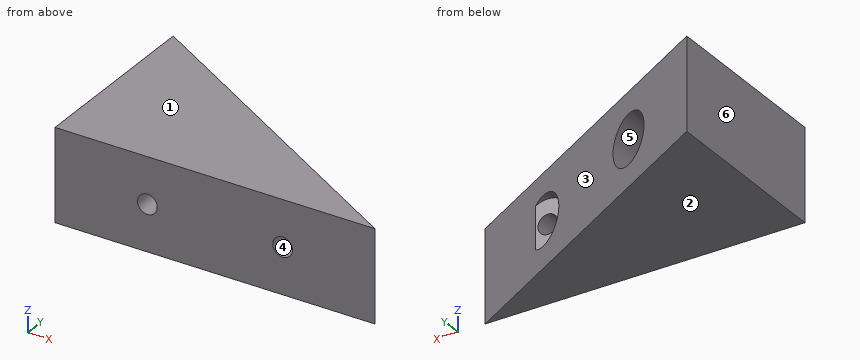
```python
from build123d import *

# Parameters (mm, degrees)
EXTRUDE_1_DEPTH          = 15
SKETCH_2_R               = 1.6
CUT_EXTRUDE_1_DEPTH      = 43.426406871
CUT_EXTRUDE_2_DEPTH      = 34.541019662
CUT_EXTRUDE_2_DEPTH_BACK = 7.5
SKETCH_3_R               = 4
SKETCH_3_R_2             = 1.6


with BuildPart() as part:
    # ｽｹｯﾁ1 → ﾎﾞｽ - 押し出し1 (new body)
    with BuildSketch(Plane.XY):
        Polygon((-25.980762114, 15), (-25.980762114, -15), (25.980762114, -15), align=None)
    extrude(amount=EXTRUDE_1_DEPTH)

    # ｽｹｯﾁ2 → ｶｯﾄ - 押し出し1 (cut, through all)
    with BuildSketch(Plane.XZ.offset(15)):
        with Locations(Location((-10.980762114, 7.5, 0), (0, 0, 270))):
            Circle(SKETCH_2_R)
        with Locations(Location((10.980762114, 7.5, 0), (0, 0, 270))):
            Circle(SKETCH_2_R)
    extrude(amount=-CUT_EXTRUDE_1_DEPTH, mode=Mode.SUBTRACT)

    # ｽｹｯﾁ3 → ｶｯﾄ - 押し出し2 (cut, two sides: drawn at the far end of the back side and taken through both)
    # profile 1 of 2: a face of its own
    with BuildSketch(Plane(origin=(0, 0, 0), x_dir=(1, 0, 0), z_dir=(0, 1, 0)).offset(-CUT_EXTRUDE_2_DEPTH_BACK)):
        with Locations((-10.980762114, -7.5)):
            Circle(SKETCH_3_R)
        with Locations(Location((-10.980762114, -7.5, 0), (0, 0, 90))):
            Circle(SKETCH_3_R_2, mode=Mode.SUBTRACT)
    # profile 2 of 2: a face of its own
    with BuildSketch(Plane(origin=(0, 0, 0), x_dir=(1, 0, 0), z_dir=(0, 1, 0)).offset(-CUT_EXTRUDE_2_DEPTH_BACK)):
        with Locations((10.980762114, -7.5)):
            Circle(SKETCH_3_R)
        with Locations(Location((10.980762114, -7.5, 0), (0, 0, 90))):
            Circle(SKETCH_3_R_2, mode=Mode.SUBTRACT)
    extrude(amount=CUT_EXTRUDE_2_DEPTH + CUT_EXTRUDE_2_DEPTH_BACK, mode=Mode.SUBTRACT)


solid = part.part
```
Check sheet for the modelled part. Datum: model origin and axes. Units: mm. Face numbers are marked on the shaded views. A direction names the side the tool comes from. Give positions to 0.01 mm unless a question says otherwise; leave off trailing zeros. Write each loop counter-clockwise with the first axis right and the second up, starting at its lowest first coordinate (ties: lowest second). Pieces come first, ordered by that corner, then holes.
Item 1: Cross-section at A-A (y = -10). Enter the section's corners in (x, z).
Item 2: Scan lines: L1, parallel to X at y = -10.5, z = 7.5; L2, parallel to X at y = -4.9, z = 7.5; L3, parallel to X at y = -11.75, z = 7.5. Record each from-to range of solid material in increasing order.
Item 3: Cross-section at D-D (x = -4.5). Enter the section's corners in (y, z), and give its area (3 significant figures).
Item 4: Access from +Z, -Z, +X, -X, +Y, -Y to the whole of each face (thin tool, end or side, straight path). Record for the marked faces 5 and 6.
Item 5: Cross-section at B-B (z = 7.5). Enter the section's corners in (x, y).
Item 6: Gauge pin test, flat ends, axial feed: pin 1 (6 mm diameter, centred on x = -5, y = -3.5, fed in from -Z); pin 2 (3 mm diameter, centred on x = 11.5, z = 6.5, fed in from +Y); pin 3 (4 mm diameter, centred on x = 1.5, z = 11, fed in from +Y). Record the tip position at first contact, or that the pin passes through.
Item 7: Cross-section at C-C (y = 2). Enter the section's corners in (x, z), and give its area (3 significant figures).
Item 8: Draft check along Z on the marked faces 1, 2, 3 and 4. Enter one of: released by +Z, released by -Z, zero draft, split by the parting line, or undercut.
Report:
1. outline: (-25.98, 0) - (17.32, 0) - (17.32, 15) - (-25.98, 15) - close; hole circle Ø3.2 at (-10.98, 7.5); hole circle Ø3.2 at (10.98, 7.5)
2. L1: x = -25.98 to -12.58, -9.38 to 9.38, 12.58 to 18.19
2. L2: x = -25.98 to -14.98, -6.98 to 6.98
2. L3: x = -25.98 to -12.58, -9.38 to 9.38, 12.58 to 20.35
3. outline: (-15, 0) - (2.6, 0) - (2.6, 15) - (-15, 15) - close
3. area: 264 mm2
4. face 5: +Y
4. face 6: +Z, -Z, -X, +Y, -Y
5. outline: (-25.98, -15) - (-12.58, -15) - (-12.58, -7.5) - (-14.98, -7.5) - (-14.98, 8.65) - (-25.98, 15) - close; (-9.38, -15) - (9.38, -15) - (9.38, -7.5) - (6.98, -7.5) - (6.98, -4.03) - (-6.98, 4.03) - (-6.98, -7.5) - (-9.38, -7.5) - close; (12.58, -15) - (25.98, -15) - (12.99, -7.5) - (12.58, -7.5) - close
6. pin 1: stops at z = 0
6. pin 2: stops at y = -7.5
6. pin 3: stops at y = 0.29
7. outline: (-25.98, 0) - (-3.46, 0) - (-3.46, 15) - (-25.98, 15) - close; hole circle Ø8 at (-10.98, 7.5)
7. area: 287 mm2
8. face 1: released by +Z
8. face 2: released by -Z
8. face 3: zero draft
8. face 4: undercut
